from build123d import *

# Parameters (mm, degrees)
F0_R     = 3
F1_DEPTH = 1.4
F0_W     = 13.5
F0_H     = 13.5
F2_DEPTH = 0.9
F4_DEPTH = 25


with BuildPart() as f1:
    # F0 (on Front) → F1 (new body)
    with BuildSketch(Plane.XZ):
        Circle(F0_R)
    extrude(amount=F1_DEPTH)

    # F0 (on Front) → F2 (join)
    with BuildSketch(Plane.XZ):
        Rectangle(F0_W, F0_H)
        Circle(F0_R, mode=Mode.SUBTRACT)
    extrude(amount=F2_DEPTH)

    # F3 (on face) → F4 (cut)
    with BuildSketch(Plane.XZ.offset(0.9)):
        with BuildLine():
            Line((6.75, 6.75), (4.7308, 6.75))
            ThreePointArc((4.7308, 6.75), (5.32221, 5.32221), (6.75, 4.7308))
            Line((6.75, 4.7308), (6.75, 6.75))
        make_face()
        with BuildLine():
            ThreePointArc((6.75, 4.7308), (8.17779, 5.32221), (8.7692, 6.75))
            ThreePointArc((8.7692, 6.75), (6.75, 8.7692), (4.7308, 6.75))
            Line((4.7308, 6.75), (6.75, 6.75))
            Line((6.75, 6.75), (6.75, 4.7308))
        make_face()
        with BuildLine():
            Line((-6.75, -6.75), (-6.75, -4.7308))
            ThreePointArc((-6.75, -4.7308), (-8.17779, -8.17779), (-4.7308, -6.75))
            Line((-4.7308, -6.75), (-6.75, -6.75))
        make_face()
        with BuildLine():
            ThreePointArc((-4.7308, -6.75), (-5.32221, -5.32221), (-6.75, -4.7308))
            Line((-6.75, -4.7308), (-6.75, -6.75))
            Line((-6.75, -6.75), (-4.7308, -6.75))
        make_face()
    extrude(amount=-F4_DEPTH, mode=Mode.SUBTRACT)


solid = f1.part
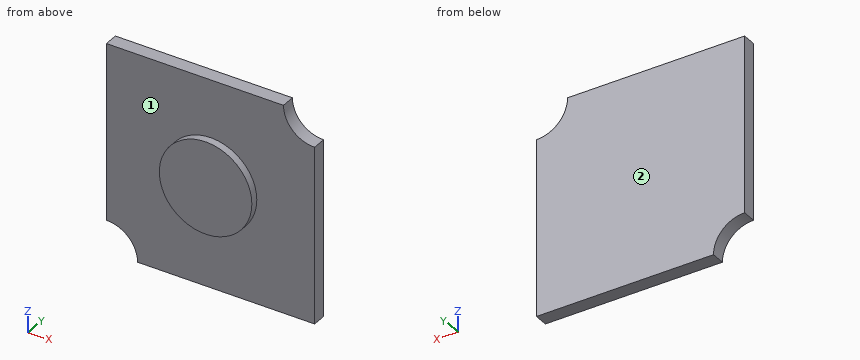
Design review of the part built by this model. Coordinates are the model's own, in mm. Face numbers are marked on the shaded views. A direction names the side the tool comes from. Round coordinates to 2 decimals unless told otherwise and drop trailing zeros. Order: outer loops, then holes, each group sorted by start corner. A loop starts at its lowest first (then second) coordinate and runs counter-clockwise, first axis right, second up.
1) Consider section B-B (z = 0). State the section outline as (x, y) points.
The answers:
outline: (-6.75, -0.9) - (-3, -0.9) - (-3, -1.4) - (3, -1.4) - (3, -0.9) - (6.75, -0.9) - (6.75, 0) - (-6.75, 0) - close
2) Clearance check with a flat-ended pin moving along its axis: pin 1 Ø2 at (x, z) = (5, 2) entering from -Y. State where the tip first meets the part, or that it passes through.
The answers:
pin 1: stops at y = -0.9
3) Machinability: for the marked faces 1 and 2, which of the approach directions +Z, -Z, +X, -X, +Y, -Y give a long, thin tool a straight path to every point of the face, cutting with its end or side? Answer none if there is none.
The answers:
face 1: -Y
face 2: +Z, -Z, +X, -X, +Y
4) Consider section A-A (x = 0). State the section outline as (y, z) points.
The answers:
outline: (-1.4, -3) - (-0.9, -3) - (-0.9, -6.75) - (0, -6.75) - (0, 6.75) - (-0.9, 6.75) - (-0.9, 3) - (-1.4, 3) - close
5) For L1, parallel to Y at x = -4.75, z = 5; L2, parallel to X at y = -0.1, z = 5.5; L3, parallel to Z at x = -1.75, y = -1.2, list the stretches that pass through material, from the lowest coordinate up.
The answers:
L1: y = -0.9 to 0
L2: x = -6.75 to 5.16
L3: z = -2.44 to 2.44
6) Consider section D-D (x = -3.5). State the section outline as (y, z) points, plus the area to 4 significant figures.
The answers:
outline: (-0.9, -6.75) - (0, -6.75) - (0, 6.75) - (-0.9, 6.75) - close
area: 12.15 mm2
7) Consider section C-C (y = -0.35). State the section outline as (x, z) points, plus the area to 3 significant figures.
The answers:
outline: (-6.75, -4.73) arc R2.02 cw to (-4.73, -6.75) - (6.75, -6.75) - (6.75, 4.73) arc R2.02 cw to (4.73, 6.75) - (-6.75, 6.75) - close
area: 176 mm2
